Geometry: final body of the model. Coordinates: model frame, mm. A direction names the side the tool comes from. Round coordinates to 2 decimals unless told otherwise and drop trailing zeros. Answer in a Markdown table with one row per item. Add a question column.
from build123d import *

# Parameters (mm, degrees)
BOSS_EXTRUDE1_DEPTH = 228.6
FILLET1_R           = 2.54
FILLET2_R           = 1.016
FILLET3_R           = 1.016


with BuildPart() as part:
    # Sketch1 → Boss-Extrude1 (new body)
    with BuildSketch(Plane.XY):
        Polygon((1.562564565, 25.4), (3.912064565, 23.0505), (9.4615, 23.0505), (9.4615, 25.4), align=None)
        with BuildLine():
            Line((11.814337736, 15.148226829), (9.754064565, 17.2085))
            Line((9.754064565, 17.2085), (3.912064565, 23.0505))
            Line((3.912064565, 23.0505), (1.562564565, 25.4))
            Line((1.562564565, 25.4), (0, 25.4))
            Line((0, 25.4), (0, 23.837435435))
            Line((0, 23.837435435), (2.3495, 21.487935435))
            Line((2.3495, 21.487935435), (8.1915, 15.645935435))
            Line((8.1915, 15.645935435), (10.251773171, 13.585662264))
            ThreePointArc((10.251773171, 13.585662264), (10.859047495, 14.540952505), (11.814337736, 15.148226829))
        make_face()
        Polygon((2.3495, 15.9385), (2.3495, 21.487935435), (0, 23.837435435), (0, 15.9385), align=None)
        with BuildLine():
            Line((13.585662264, 15.148226829), (15.645935435, 17.2085))
            Line((15.645935435, 17.2085), (9.754064565, 17.2085))
            Line((9.754064565, 17.2085), (11.814337736, 15.148226829))
            ThreePointArc((11.814337736, 15.148226829), (12.7, 15.3035), (13.585662264, 15.148226829))
        make_face()
        with BuildLine():
            ThreePointArc((10.251773171, 11.814337736), (10.0965, 12.7), (10.251773171, 13.585662264))
            Line((10.251773171, 13.585662264), (8.1915, 15.645935435))
            Line((8.1915, 15.645935435), (8.1915, 9.754064565))
            Line((8.1915, 9.754064565), (10.251773171, 11.814337736))
        make_face()
        with BuildLine():
            ThreePointArc((11.814337736, 10.251773171), (10.859047495, 10.859047495), (10.251773171, 11.814337736))
            Line((10.251773171, 11.814337736), (8.1915, 9.754064565))
            Line((8.1915, 9.754064565), (2.3495, 3.912064565))
            Line((2.3495, 3.912064565), (0, 1.562564565))
            Line((0, 1.562564565), (0, 0))
            Line((0, 0), (1.562564565, 0))
            Line((1.562564565, 0), (3.912064565, 2.3495))
            Line((3.912064565, 2.3495), (9.754064565, 8.1915))
            Line((9.754064565, 8.1915), (11.814337736, 10.251773171))
        make_face()
        with BuildLine():
            ThreePointArc((13.585662264, 10.251773171), (12.7, 10.0965), (11.814337736, 10.251773171))
            Line((11.814337736, 10.251773171), (9.754064565, 8.1915))
            Line((9.754064565, 8.1915), (15.645935435, 8.1915))
            Line((15.645935435, 8.1915), (13.585662264, 10.251773171))
        make_face()
        with BuildLine():
            Line((17.2085, 9.754064565), (15.148226829, 11.814337736))
            ThreePointArc((15.148226829, 11.814337736), (14.540952505, 10.859047495), (13.585662264, 10.251773171))
            Line((13.585662264, 10.251773171), (15.645935435, 8.1915))
            Line((15.645935435, 8.1915), (21.487935435, 2.3495))
            Line((21.487935435, 2.3495), (23.837435435, 0))
            Line((23.837435435, 0), (25.4, 0))
            Line((25.4, 0), (25.4, 1.562564565))
            Line((25.4, 1.562564565), (23.0505, 3.912064565))
            Line((23.0505, 3.912064565), (17.2085, 9.754064565))
        make_face()
        with BuildLine():
            Line((17.2085, 15.645935435), (15.148226829, 13.585662264))
            ThreePointArc((15.148226829, 13.585662264), (15.264387919, 13.149585199), (15.3035, 12.7))
            ThreePointArc((15.3035, 12.7), (15.264387919, 12.250414801), (15.148226829, 11.814337736))
            Line((15.148226829, 11.814337736), (17.2085, 9.754064565))
            Line((17.2085, 9.754064565), (17.2085, 15.645935435))
        make_face()
        with BuildLine():
            Line((23.837435435, 25.4), (21.487935435, 23.0505))
            Line((21.487935435, 23.0505), (15.645935435, 17.2085))
            Line((15.645935435, 17.2085), (13.585662264, 15.148226829))
            ThreePointArc((13.585662264, 15.148226829), (14.540952505, 14.540952505), (15.148226829, 13.585662264))
            Line((15.148226829, 13.585662264), (17.2085, 15.645935435))
            Line((17.2085, 15.645935435), (23.0505, 21.487935435))
            Line((23.0505, 21.487935435), (25.4, 23.837435435))
            Line((25.4, 23.837435435), (25.4, 25.4))
            Line((25.4, 25.4), (23.837435435, 25.4))
        make_face()
        Polygon((15.9385, 23.0505), (21.487935435, 23.0505), (23.837435435, 25.4), (15.9385, 25.4), align=None)
        Polygon((25.4, 15.9385), (25.4, 23.837435435), (23.0505, 21.487935435), (23.0505, 15.9385), align=None)
        Polygon((23.0505, 9.4615), (23.0505, 3.912064565), (25.4, 1.562564565), (25.4, 9.4615), align=None)
        Polygon((23.837435435, 0), (21.487935435, 2.3495), (15.9385, 2.3495), (15.9385, 0), align=None)
        Polygon((9.4615, 2.3495), (3.912064565, 2.3495), (1.562564565, 0), (9.4615, 0), align=None)
        Polygon((0, 1.562564565), (2.3495, 3.912064565), (2.3495, 9.4615), (0, 9.4615), align=None)
    extrude(amount=BOSS_EXTRUDE1_DEPTH)

    # Fillet1
    fillet1_edges = [part.edges().sort_by_distance(p)[0] for p in [
        (15.645935435, 8.1915, 114.3),
        (9.754064565, 8.1915, 114.3),
        (8.1915, 9.754064565, 114.3),
        (8.1915, 15.645935435, 114.3),
        (9.754064565, 17.2085, 114.3),
        (15.645935435, 17.2085, 114.3),
        (17.2085, 15.645935435, 114.3),
        (17.2085, 9.754064565, 114.3),
    ]]
    fillet(fillet1_edges, radius=FILLET1_R)

    # Fillet2
    fillet2_edges = [part.edges().sort_by_distance(p)[0] for p in [
        (23.0505, 9.4615, 114.3),
        (25.4, 9.4615, 114.3),
        (25.4, 0, 114.3),
        (15.9385, 0, 114.3),
        (15.9385, 2.3495, 114.3),
        (9.4615, 2.3495, 114.3),
        (9.4615, 0, 114.3),
        (0, 0, 114.3),
        (0, 9.4615, 114.3),
        (2.3495, 9.4615, 114.3),
        (2.3495, 15.9385, 114.3),
        (0, 15.9385, 114.3),
        (0, 25.4, 114.3),
        (9.4615, 25.4, 114.3),
        (9.4615, 23.0505, 114.3),
        (15.9385, 23.0505, 114.3),
        (15.9385, 25.4, 114.3),
        (25.4, 25.4, 114.3),
        (25.4, 15.9385, 114.3),
        (23.0505, 15.9385, 114.3),
    ]]
    fillet(fillet2_edges, radius=FILLET2_R)

    # Fillet3
    fillet3_edges = [part.edges().sort_by_distance(p)[0] for p in [
        (23.0505, 3.912064565, 114.3),
        (21.487935435, 2.3495, 114.3),
        (3.912064565, 2.3495, 114.3),
        (2.3495, 3.912064565, 114.3),
        (2.3495, 21.487935435, 114.3),
        (3.912064565, 23.0505, 114.3),
        (21.487935435, 23.0505, 114.3),
        (23.0505, 21.487935435, 114.3),
    ]]
    fillet(fillet3_edges, radius=FILLET3_R)


solid = part.part
1) Reachability of faces 5 (the flat face through (8.192, 13, 113)), 6 (the flat face through (0, 21, 113)), 7 (the flat face through (13, 17.208, 113)) from +Z, -Z, +X, -X, +Y, -Y: full face, straight path, thin tool, end or side. Return the list, or none.
2) Contact query for flat-ended pins moving along their axis: pin 1 Ø1.1 at (y, z) = (12.5, 100) entering from -X; pin 2 Ø4 at (x, z) = (12.5, 137.5) entering from -Y; pin 3 Ø1.9 at (y, z) = (12.5, 165.5) entering from +X. Output: stop coordinate, or through.
3) Material intervals for line 1 along Y through (x, z) = (18.5, 22.5); line 2 along X through (y, z) = (22.75, 61); line 3 along Y through (x, z) = (17.5, 102), sorted ascending. Write a range as from..to.
4) Pull-direction query (Y, two-part tool) for faces 1 (the flat face through (25.4, 21, 113)), 2 (the flat face through (5, 25.4, 113)), 3 (the flat face through (17.208, 13, 113)), 4 (the flat face through (13, 8.192, 113)); classes: pulls with the +Y half, pulls with the -Y half, needs draft (parallel to the pull), parting line crosses it, or undercut.
Evaluation:
| question | item | result |
|---|---|---|
| 1 | face 5 | +Z, -Z, -X |
| 1 | face 6 | +Z, -Z, -X, +Y, -Y |
| 1 | face 7 | +Z, -Z, +Y |
| 2 | pin 1 | stops at x = 8.19 |
| 2 | pin 2 | stops at y = 8.17 |
| 2 | pin 3 | stops at x = 17.21 |
| 3 | line 1 | y = 0..2.35, 5.34..8.46, 16.94..20.06, 23.05..25.4 |
| 3 | line 2 | x = 0..5.64, 19.76..25.4 |
| 3 | line 3 | y = 0..2.35, 6.34..9.62, 15.78..19.06, 23.05..25.4 |
| 4 | face 1 | needs draft |
| 4 | face 2 | pulls with the +Y half |
| 4 | face 3 | undercut |
| 4 | face 4 | pulls with the -Y half |
